Source: CAD feature listing. Evaluate the final solid. Frame: model axes, mm. Give positions to 0.01 mm unless a question says otherwise; leave off trailing zeros. Loops run counter-clockwise (first coordinate to the right, second up) from the corner with the lowest first, then second, coordinate; pieces in that order, holes last. Notation, with made-up numbers: M 36.25,40 L 41.25,40 A16 cw 41.25,66 Z; hole C 1,71 d3. An arc over 180 degrees is marked long. Put each result on its own line as item: value.
from build123d import *

# Parameters (mm, degrees)
SKETCH_1_R             = 10
EXTRUDE_1_DEPTH        = 200
CUT_EXTRUDE_1_DEPTH    = 3
CHAMFER_1_SIZE         = 1
CHAMFER_2_SIZE         = 1
PATTERN_LINEAR_1_COUNT = 3
PATTERN_LINEAR_1_PITCH = 80
CUT_EXTRUDE_START      = -40
SKETCH_4_R             = 10
CUT_EXTRUDE_2_DEPTH    = 40
PATTERN_LINEAR_3_COUNT = 2
PATTERN_LINEAR_3_PITCH = 125


with BuildPart() as part:
    # 草图1 → 凸台-拉伸1 (new body)
    with BuildSketch(Plane(origin=(0, 0, 0), x_dir=(0, 0, -1), z_dir=(1, 0, 0))):
        Circle(SKETCH_1_R)
    extrude(amount=EXTRUDE_1_DEPTH)

    # 草图2 → 切除-拉伸1 (cut)
    with BuildSketch(Plane(origin=(0, 10, 0), x_dir=(1, 0, 0), z_dir=(0, 1, 0))):
        with BuildLine():
            Line((13, 3), (27, 3))
            ThreePointArc((27, 3), (30, 0), (27, -3))
            Line((27, -3), (13, -3))
            ThreePointArc((13, -3), (10, 0), (13, 3))
        make_face()
    cut_extrude_1 = extrude(amount=-CUT_EXTRUDE_1_DEPTH, mode=Mode.SUBTRACT)

    # 倒角1
    chamfer_1_edges = [part.edges().sort_by_distance(p)[0] for p in [
        (0, 0, 10),
    ]]
    chamfer(chamfer_1_edges, length=CHAMFER_1_SIZE)

    # 倒角2
    chamfer_2_edges = [part.edges().sort_by_distance(p)[0] for p in [
        (200, 0, 10),
    ]]
    chamfer(chamfer_2_edges, length=CHAMFER_2_SIZE)

    # 阵列(线性)1: 切除-拉伸1 ×3
    with Locations(*[(i * PATTERN_LINEAR_1_PITCH, 0, 0) for i in range(1, PATTERN_LINEAR_1_COUNT)]):
        add(cut_extrude_1, mode=Mode.SUBTRACT)

    # 草图4 → 切除-拉伸2 (cut)
    with BuildSketch(Plane(origin=(200, 0, 0), x_dir=(0, 0, -1), z_dir=(1, 0, 0)).offset(CUT_EXTRUDE_START)):
        Circle(SKETCH_4_R)
    extrude(amount=CUT_EXTRUDE_2_DEPTH, mode=Mode.SUBTRACT)

    # 阵列(线性)3: 切除-拉伸1 ×2
    with Locations(*[(i * PATTERN_LINEAR_3_PITCH, 0, 0) for i in range(1, PATTERN_LINEAR_3_COUNT)]):
        add(cut_extrude_1, mode=Mode.SUBTRACT)


solid = part.part
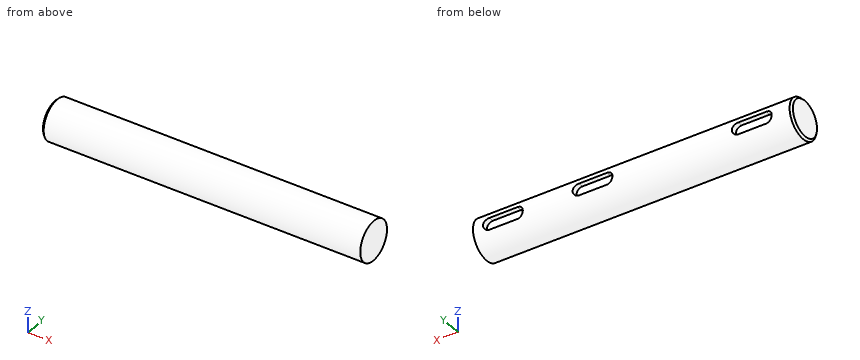
1. Section query C-C (x = 19). Output: boundary loops of the cut face in (y, z), plus the area to 3 significant figures.
Found:
outline: M 7,-3 L 7,3 L 9.54,3 A10 ccw long 9.54,-3 Z
area: 297 mm^2
2. Section query A-A (z = 0). Output: boundary loops of the cut face in (x, y).
Found:
outline: M 0,-9 L 1,-10 L 160,-10 L 160,10 L 155,10 L 155,7 L 135,7 L 135,10 L 110,10 L 110,7 L 90,7 L 90,10 L 30,10 L 30,7 L 10,7 L 10,10 L 1,10 L 0,9 Z
3. Contact query for flat-ended pins moving along their axis: P1, Ø2, axis at x = 98, y = 8, coming from the +Z side; P2, Ø3, axis at x = 98, y = 7.5, coming from the -Z side; P3, Ø1, axis at x = 91.5, y = 1, coming from the +Z side. Output: stop coordinate, or through.
Found:
P1: z = 7.14
P2: z = -8
P3: z = 9.99
4. Material intervals for line 1 (Y direction, x = 15.5, z = -0.5); line 2 (Z direction, x = 18.5, y = 0.5); line 3 (Z direction, x = 49.5, y = -1.5), sorted ascending. Write a range as from..to.
Found:
line 1: -9.99..7
line 2: -9.99..9.99
line 3: -9.89..9.89
5. Section query B-B (x = 76.5). Output: boundary loops of the cut face in (y, z), plus the area to 3 significant figures.
Found:
outline: C 0,0 d20
area: 314 mm^2
